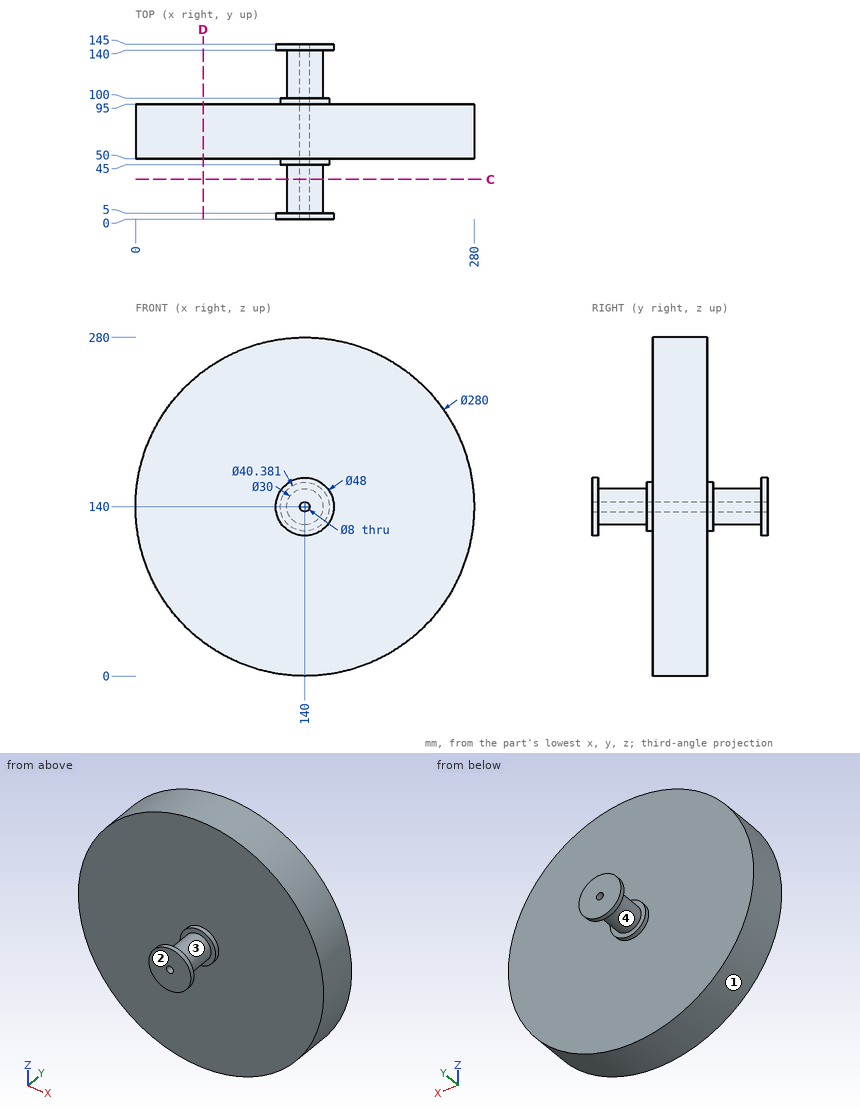
Drawing for the job (mm, zero at the part's lowest x, y, z). Give positions to 0.01 mm unless a question says otherwise; leave off trailing zeros. Loops run counter-clockwise (first coordinate to the right, second up) from the corner with the lowest first, then second, coordinate; pieces in that order, holes last.
Item 1: Drop flat-ended pins along their axis: P1, Ø12, axis at y = 113, z = 147.5, coming from the +X side; P2, Ø1, axis at y = 72, z = 155, coming from the +X side; P3, Ø2, axis at x = 33.5, z = 184.5, coming from the -Y side. Give the stop position or say it passes through.
Check values:
P1: stops at x = 154.92
P2: stops at x = 279.25
P3: stops at y = 50
Item 2: Drill centre lines: line 1 along Y through (x, z) = (145.5, 125); line 2 along X through (y, z) = (102.5, 140); line 3 along X through (y, z) = (70, 140). Where is each one in solid material? Low to high.
Check values:
line 1: y = 0 to 5, 45 to 100, 140 to 145
line 2: x = 125 to 136, 144 to 155
line 3: x = 0 to 136, 144 to 280
Item 3: Mould opens along Y. For the marked faces 1, 2, 3 and 4 say: +Y half, -Y half, draft (parallel to the pull), parting line (faces both ways), or undercut.
Check values:
face 1: draft
face 2: -Y half
face 3: undercut
face 4: undercut
Item 4: Slice it at D-D (x = 56). Write the cut outline in (y, z).
Check values:
outline: (50, 28) - (95, 28) - (95, 252) - (50, 252) - close
Item 5: Slice it at C-C (y = 33). Write the cut outline in (x, z).
Check values:
outline: circle Ø30 at (140, 140); hole circle Ø8 at (140, 140)
